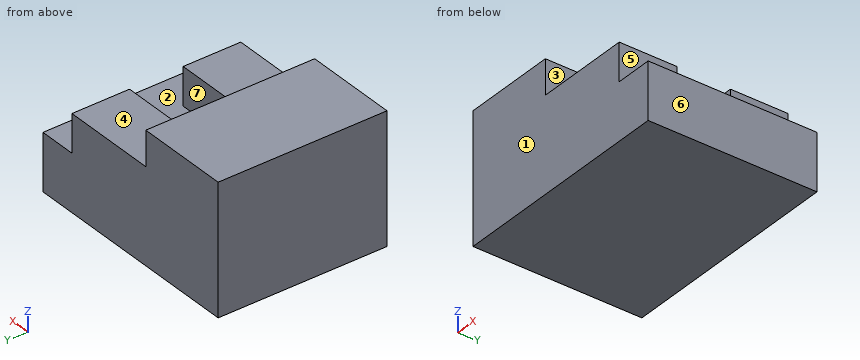
from build123d import *

# Parameters (mm, degrees)
F0_W      = 58.42
F0_H      = 43.18
F1_DEPTH  = 33.02
F2_W      = 44.949538
F2_H      = 18.542
F3_DEPTH  = 21.591
F3_FACE_W = 34.29
F3_FACE_H = 18.542
F4_DEPTH  = 21.591
F5_W      = 24.638
F5_H      = 14.732
F6_DEPTH  = 24.13
F7_W      = 24.638
F7_H      = 14.732
F8_DEPTH  = 24.13


with BuildPart() as f1:
    # F0 (on Top) → F1 (new body)
    with BuildSketch(Plane.XY):
        Rectangle(F0_W, F0_H)
    extrude(amount=F1_DEPTH)

    # F2 (on Front) → F3 (cut, through all)
    with BuildSketch(Plane.XZ):
        with Locations((17.394769, 23.749)):
            Rectangle(F2_W, F2_H)
    extrude(amount=-F3_DEPTH, mode=Mode.SUBTRACT)

    # F3_face (on face) → F4 (cut, through all)
    with BuildSketch(Plane(origin=(12.065, 0, 23.749), x_dir=(1, 0, 0), z_dir=(0, 1, 0))):
        Rectangle(F3_FACE_W, F3_FACE_H)
    extrude(amount=-F4_DEPTH, mode=Mode.SUBTRACT)

    # F5 (on Top) → F6 (join)
    with BuildSketch(Plane.XY):
        with Locations((7.239, 14.224)):
            Rectangle(F5_W, F5_H)
    extrude(amount=F6_DEPTH)

    # F7 (on Top) → F8 (join)
    with BuildSketch(Plane.XY):
        with Locations((7.239, -14.224)):
            Rectangle(F7_W, F7_H)
    extrude(amount=F8_DEPTH)


solid = f1.part
The model under review builds one solid part; all positions refer to its coordinate system, in mm. Face numbers are marked on the shaded views. A direction names the side the tool comes from. Round coordinates to 2 decimals unless told otherwise and drop trailing zeros. Order: outer loops, then holes, each group sorted by start corner. A loop starts at its lowest first (then second) coordinate and runs counter-clockwise, first axis right, second up. Notation, with made-up numbers: (-20.75, -36) -> (30.25, -36) arc R13 ccw to (30.25, -27) -> close; hole circle Ø8 at (66, 27). An arc over 180 degrees is marked (long way). Write item = value, one per line. Start each with the question number.
Item 1: For the marked faces 5, 6 and 7, list the 3-axis set-ups (+Z, -Z, +X, -X, +Y, -Y) from which the entire face can be reached by the end or side of a thin tool; tool diameter is ignored.
Item 2: Consider section C-C on y = 1. Write out the cut boundary in (x, z), plus the area to 3 significant figures.
Item 3: Consider section D-D on z = 29. Write out the cut boundary in (x, y), plus the area to 3 significant figures.
Item 4: Consider section B-B on z = 18.5. Write out the cut boundary in (x, y).
Item 5: Consider section A-A on y = 12.5. Write out the cut boundary in (x, z), plus the area to 3 significant figures.
Item 6: For line 1 along Z through (x, y) = (21.5, 18); line 2 along X through (y, z) = (-7.5, 27.5); line 3 along Z through (x, y) = (-4, 7.5), list the stretches that pass through material, from the lowest coordinate up.
Item 7: Clearance check with flat-ended pins moving along their axes: pin 1 Ø1 at (x, y) = (21, -2.5) entering from +Z; pin 2 Ø4.5 at (x, y) = (2.5, -11.5) entering from +Z; pin 3 Ø5 at (y, z) = (12, 18.5) entering from +X; pin 4 Ø5 at (x, y) = (9, -16.5) entering from -Z. State where each tip first meets the part, or that it passes through.
Item 8: Mouldability with a two-part tool opening along Y and no side actions: class the marked faces 1, 2, 3 and 4 as released by +Y, released by -Y, zero draft, split by the parting line, or undercut.
Conclusion:
q1.face_5 = +Z, +X, +Y, -Y
q1.face_6 = +Z, -Z, +X, +Y, -Y
q1.face_7 = +Z, +X
q2.outline = (-29.21, 0) -> (29.21, 0) -> (29.21, 14.48) -> (-5.08, 14.48) -> (-5.08, 33.02) -> (-29.21, 33.02) -> close
q2.area = 1,290 mm2
q3.outline = (-29.21, -21.59) -> (-5.08, -21.59) -> (-5.08, 21.59) -> (-29.21, 21.59) -> close
q3.area = 1,040 mm2
q4.outline = (-29.21, -21.59) -> (19.56, -21.59) -> (19.56, -6.86) -> (-5.08, -6.86) -> (-5.08, 6.86) -> (19.56, 6.86) -> (19.56, 21.59) -> (-29.21, 21.59) -> close
q5.outline = (-29.21, 0) -> (29.21, 0) -> (29.21, 14.48) -> (19.56, 14.48) -> (19.56, 24.13) -> (-5.08, 24.13) -> (-5.08, 33.02) -> (-29.21, 33.02) -> close
q5.area = 1,530 mm2
q6.line_1 = 0 to 14.48
q6.line_2 = -29.21 to -5.08
q6.line_3 = 0 to 24.13
q7.pin_1 = 14.48
q7.pin_2 = 24.13
q7.pin_3 = 19.56
q7.pin_4 = 0
q8.face_1 = released by -Y
q8.face_2 = undercut
q8.face_3 = undercut
q8.face_4 = zero draft
